Geometry: final body of the model. Coordinates: model frame, mm. Give positions to 0.01 mm unless a question says otherwise; leave off trailing zeros. Order: outer loops, then holes, each group sorted by start corner. A loop starts at its lowest first (then second) coordinate and runs counter-clockwise, first axis right, second up. Notation, with made-up numbers: (72.25, 29) - (125.25, 29) arc R23 ccw to (125.25, 43) - close; hole circle Ø1 at (-8.5, 83). An arc over 180 degrees is marked (long way). Write item = value, one per line. Start each with the question number.
from build123d import *

# Parameters (mm, degrees)
SKETCH1_W           = 400
SKETCH1_H           = 225
BOSS_EXTRUDE1_DEPTH = 18
SWEEP1_OUTLINE_R    = 5
SWEEP1_ANGLE        = 180


# Read off the part's stored shape, not the designer's step: Sweep1
with BuildPart() as part:
    # Sketch1 → Boss-Extrude1 (new body)
    with BuildSketch(Plane.XY):
        with Locations((200, 112.5)):
            Rectangle(SKETCH1_W, SKETCH1_H)
    extrude(amount=BOSS_EXTRUDE1_DEPTH)

    # Sweep1 outline → Sweep1 (revolve)
    with BuildSketch(Plane(origin=(200, 0, 18), x_dir=(-1, 0, 0), z_dir=(0, 0, -1))):
        with Locations((60, 112.5)):
            Circle(SWEEP1_OUTLINE_R)
    revolve(axis=Axis((200, 0, 18), (0, 1, 0)), revolution_arc=SWEEP1_ANGLE)


solid = part.part
Q1. Contact query for a flat-ended pin moving along its axis: pin 1 (2 mm diameter, centred on x = 257, y = 161, fed in from +Z). Output: stop coordinate, or through.
Q2. Material intervals for line 1 along Z through (x, y) = (206, 32.5); line 2 along X through (y, z) = (116.5, 47); line 3 along Y through (x, z) = (189, 77), sorted ascending. Write a range as from..to.
Q3. Section B-B, the plane x = 276.5. Return the cut outline in (y, z).
Q4. Section A-A, the plane y = 69. Return the cut outline in (x, z), then the cut area to 3 significant figures.
The answers:
q1.pin_1 = 18
q2.line_1 = 0..18
q2.line_2 = 144.07..150.93, 249.07..255.93
q2.line_3 = 107.5..117.5
q3.outline = (0, 0) - (225, 0) - (225, 18) - (0, 18) - close
q4.outline = (0, 0) - (400, 0) - (400, 18) - (0, 18) - close
q4.area = 7,200 mm²
